```python
from build123d import *

# Parameters (mm, degrees)
F0_R     = 10
F1_DEPTH = 5
F2_DEPTH = 25
F4_D     = 6.5
F4_DEPTH = 12.001
F6_D     = 6.5


with BuildPart() as f1:
    # F0 (on Top) → F1 (new body)
    with BuildSketch(Plane.XY):
        with BuildLine():
            ThreePointArc((5, -12), (10.8166538264, -7.2111025509), (13, 0))
            ThreePointArc((13, 0), (10.8166538264, 7.2111025509), (5, 12))
            Line((5, 12), (-5, 12))
            ThreePointArc((-5, 12), (-13, 0), (-5, -12))
            Line((-5, -12), (5, -12))
        make_face()
        Circle(F0_R, mode=Mode.SUBTRACT)
        Circle(F0_R)
    extrude(amount=F1_DEPTH)

    # F0 (on Top) → F2 (join)
    with BuildSketch(Plane.XY):
        with BuildLine():
            ThreePointArc((5, -12), (10.8166538264, -7.2111025509), (13, 0))
            ThreePointArc((13, 0), (10.8166538264, 7.2111025509), (5, 12))
            Line((5, 12), (-5, 12))
            ThreePointArc((-5, 12), (-13, 0), (-5, -12))
            Line((-5, -12), (5, -12))
        make_face()
        Circle(F0_R, mode=Mode.SUBTRACT)
    extrude(amount=F2_DEPTH)

    # F4 (through all, one way)
    with BuildSketch(Plane.XZ):
        with Locations((0, 10)):
            Circle(F4_D / 2)
    extrude(amount=-F4_DEPTH, mode=Mode.SUBTRACT)

    # F6 (through all)
    with Locations(Plane(origin=(0, 0, 0), x_dir=(1, 0, 0), z_dir=(0, 1, 0))):
        with Locations((0, -10)):
            Hole(F6_D / 2)


solid = f1.part
```
For this review, take the finished solid that the model builds, in its own axes (mm). A direction names the side the tool comes from. Coordinates: 2 decimals unless noted, no trailing zeros. Order: outer loops, then holes, each group sorted by start corner. A loop starts at its lowest first (then second) coordinate and runs counter-clockwise, first axis right, second up. Notation, with made-up numbers: (-35.5, 42) -> (-13.5, 42) arc R28 cw to (-13.5, 74) -> close; hole circle Ø11 at (-25, 8). An arc over 180 degrees is marked (long way). Answer as CSV lines item,"result".
Q1. Clearance check with flat-ended pins moving along their axes: pin 1 Ø1.5 at (y, z) = (3.5, 15) entering from +X; pin 2 Ø4 at (y, z) = (8, 22) entering from -X; pin 3 Ø1.5 at (x, z) = (6, 18.5) entering from -Y. State where each tip first meets the part, or that it passes through.
Model answer:
pin 1,"stops at x = 12.71"
pin 2,"stops at x = -11.53"
pin 3,"stops at y = -11.89"
Q2. We need section C-C (y = 0). State the section outline as (x, z) points.
Model answer:
outline,"(-13, 0) -> (13, 0) -> (13, 25) -> (10, 25) -> (10, 5) -> (-10, 5) -> (-10, 25) -> (-13, 25) -> close"
Q3. We need section B-B (z = 10). State the section outline as (x, y) points, plus the area to 3 significant figures.
Model answer:
outline,"(-5, -12) -> (-3.25, -12) -> (-3.25, -9.46) arc R10 cw to (-3.25, 9.46) -> (-3.25, 12) -> (-5, 12) arc R13 ccw to start; (3.25, -12) -> (5, -12) arc R13 ccw to (5, 12) -> (3.25, 12) -> (3.25, 9.46) arc R10 cw to (3.25, -9.46) -> close"
area,"175 mm2"
Q4. For faces 1 (the face through (0, 0, 5)), 2 (the face through (0, 0, 0)), list the 3-axis set-ups (+Z, -Z, +X, -X, +Y, -Y) from which the entire face can be reached by the end or side of a thin tool; tool diameter is ignored.
Model answer:
face 1,"+Z"
face 2,"-Z, +X, -X, +Y, -Y"
Q5. Wall thickness on line 1 along Z through (x, y) = (0, 10.4); line 2 along X through (y, z) = (0, 10); line 3 along Z through (x, y) = (0.75, 1.25): over which ranges is each line inside the solid? List them lowest first. Write a range as [from, to].
Model answer:
line 1,"z = [0, 6.75], [13.25, 25]"
line 2,"x = [-13, -10], [10, 13]"
line 3,"z = [0, 5]"
Q6. We need section A-A (x = 0). State the section outline as (y, z) points.
Model answer:
outline,"(-12, 0) -> (12, 0) -> (12, 6.75) -> (10, 6.75) -> (10, 5) -> (-10, 5) -> (-10, 6.75) -> (-12, 6.75) -> close; (-12, 13.25) -> (-10, 13.25) -> (-10, 25) -> (-12, 25) -> close; (10, 13.25) -> (12, 13.25) -> (12, 25) -> (10, 25) -> close"
Q7. Draft analysis for pull direction Z (two halves, no side actions). For faces 3 (the face through (0, 12, 15)), 4 (the face through (-3.1, -10.74, 9.02)), 5 (the face through (-5, -9, 25)), state which applies: released by +Z, released by -Z, zero draft, split by the parting line, or undercut.
Model answer:
face 3,"zero draft"
face 4,"undercut"
face 5,"released by +Z"
Q8. We need section D-D (z = 14). State the section outline as (x, y) points.
Model answer:
outline,"(-5, -12) -> (5, -12) arc R13 ccw to (5, 12) -> (-5, 12) arc R13 ccw to start; hole circle Ø20 at (0, 0)"
